Answer from the drawing. Dimensions are ordinates in mm from the lowest x, y and z of the part. Round coordinates to 2 decimals unless told otherwise and drop trailing zeros. Loops run counter-clockwise (first coordinate to the right, second up) from the corner with the lowest first, then second, coordinate; pieces in that order, holes last. Notation, with made-up numbers: (-33, -24) - (11, -24) arc R22 cw to (11, 1) - close; hole circle Ø3 at (72.5, -32). An arc over 180 degrees is marked (long way). Write item = value, one per line. Start each with the question number.
1) Section D-D, the plane z = 60.5 is taken. Determine the outline of the cut face in (x, y) (1 decimal).
2) Straight lines are drawn through the part: line 1 along X through (y, z) = (8, 93) (1 decimal); line 2 along Z through (x, y) = (167.5, 11); line 3 along Z through (x, y) = (81.5, 6.75). For each, find the intervals that lie inside material, in ascending order.
3) For a pull along X with two mould halves and no side action, classify the marked faces 1 and 2 as released by +X, released by -X, zero draft, split by the parting line, or undercut.
4) Given pin 1 Ø2.5 at (y, z) = (10.5, 94) entering from -X; pin 2 Ø2.5 at (x, y) = (45, 8) entering from -Z; pin 3 Ø4 at (y, z) = (8, 75.5) entering from +X, each flat-ended and moving along its own axis, determine where each tip first touches the part or whether it passes through.
5) Section B-B, the plane x = 147 is taken. Determine the outline of the cut face in (y, z).
6) Section A-A, the plane z = 40 is taken. Determine the outline of the cut face in (x, y) (1 decimal).
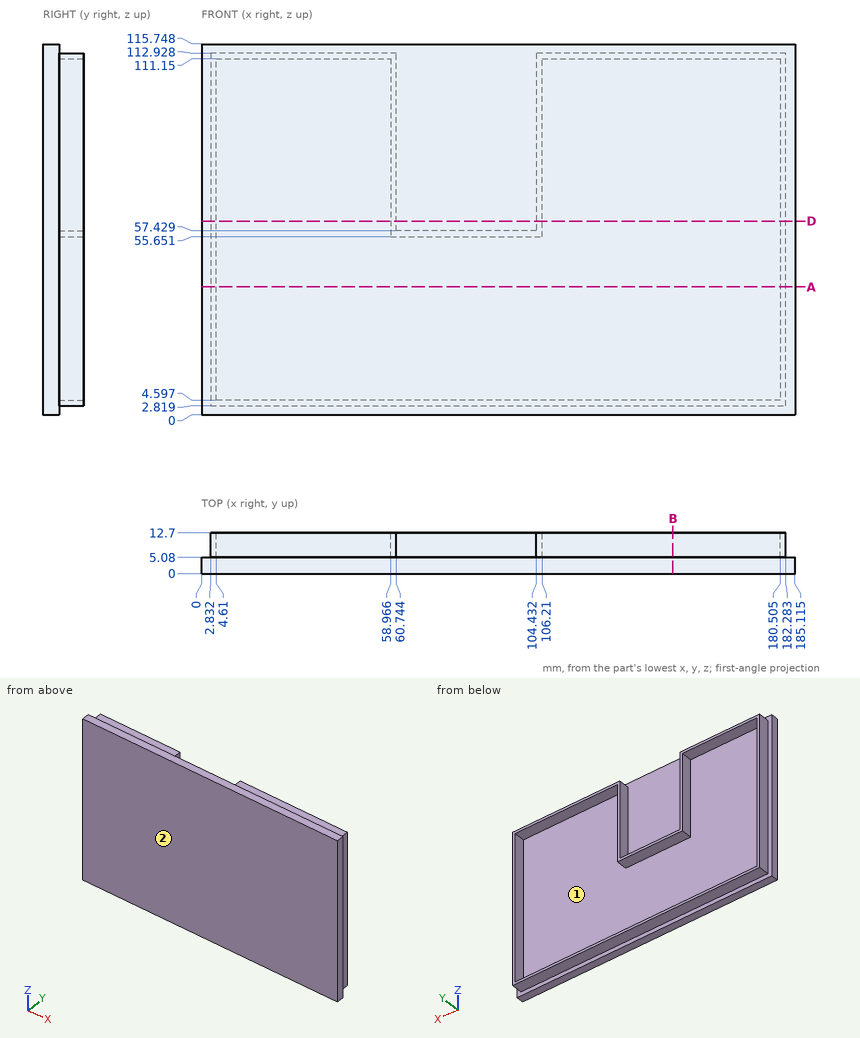
Geometry check:
q1.outline = (0, 0) - (185.1, 0) - (185.1, 5.1) - (182.3, 5.1) - (182.3, 12.7) - (180.5, 12.7) - (180.5, 5.1) - (106.2, 5.1) - (106.2, 12.7) - (104.4, 12.7) - (104.4, 5.1) - (60.7, 5.1) - (60.7, 12.7) - (59, 12.7) - (59, 5.1) - (4.6, 5.1) - (4.6, 12.7) - (2.8, 12.7) - (2.8, 5.1) - (0, 5.1) - close
q2.line_1 = 2.8 to 4.6, 59 to 60.7, 104.4 to 106.2, 180.5 to 182.3
q2.line_2 = 2.82 to 4.6, 111.15 to 112.93
q2.line_3 = 2.82 to 4.6, 55.65 to 57.43
q3.face_1 = undercut
q3.face_2 = zero draft
q4.pin_1 = 2.83
q4.pin_2 = 2.82
q4.pin_3 = 182.28
q5.outline = (0, 0) - (5.08, 0) - (5.08, 2.82) - (12.7, 2.82) - (12.7, 4.6) - (5.08, 4.6) - (5.08, 111.15) - (12.7, 111.15) - (12.7, 112.93) - (5.08, 112.93) - (5.08, 115.75) - (0, 115.75) - close
q6.outline = (0, 0) - (185.1, 0) - (185.1, 5.1) - (182.3, 5.1) - (182.3, 12.7) - (180.5, 12.7) - (180.5, 5.1) - (4.6, 5.1) - (4.6, 12.7) - (2.8, 12.7) - (2.8, 5.1) - (0, 5.1) - close
